Autodesk Fusion 360 part; units mm, degrees
sketch "Sketch1" plane through (0, 0, 0) normal (0, 0, 1) x (1, 0, 0)
  line L0 (0, 6.5) -> (0, -6.5) construction
  circle A0 centre (0, 6.5) radius 1.75
  circle A1 centre (0, -6.5) radius 1.75
  line L1 (4, -4.5) -> (-4, -4.5)
  line L2 (-4, -4.5) -> (-4, 4.5) construction
  line L3 (-4, 4.5) -> (4, 4.5)
  line L4 (4, 4.5) -> (4, -4.5) construction
  line L5 (4, -4.5) -> (-4, 4.5) construction
  line L6 (-4, -4.5) -> (4, 4.5) construction
  line L7 (4, -10.5) -> (-4, -10.5)
  line L8 (-4, -10.5) -> (-4, 10.5)
  line L9 (-4, 10.5) -> (4, 10.5)
  line L10 (4, 10.5) -> (4, -10.5)
  line L11 (4, -10.5) -> (-4, 10.5) construction
  line L12 (-4, -10.5) -> (4, 10.5) construction
  circle A2 centre (0, -6.5) radius 1.4
  circle A3 centre (0, 6.5) radius 1.4
  dimension "d1" = 13
  dimension "d2" = 3.5
  dimension "d3" = 3.5
  dimension "d5" = 9
  dimension "d10" = 2.8
  dimension "d11" = 2.8
  dimension "d14" = 4
  dimension "d15" = 4
extrude "Extrude1" add sketch "Sketch1" along normal blind 3.5 contours L1 L7 L8 L10 | L1 L3 L8 L10 | L3 L8 L9 L10
extrude "Extrude2" add sketch "Sketch1" along normal blind 1 contours A0 | A1
extrude "Extrude3" add sketch "Sketch1" along normal blind 10 contours L1 L3 L8 L10
sketch "Sketch2" plane through (0, -4.5, 0) normal (0, -1, 0) x (1, 0, 0)
  line L0 (-4, 3.5) -> (4, 3.5)
  line L1 (4, 3.5) -> (4, 10)
  line L2 (4, 10) -> (-4, 10)
  line L3 (-4, 10) -> (-4, 3.5)
  circle A0 centre (0, 6) radius 2.1
  line L4 (0, 6) -> (0, 3.5)
  circle A1 centre (0, 6) radius 1.6
  dimension "d18" = 4.2
  dimension "d19" = 2.5
  dimension "d24" = 3.2
extrude "Extrude4" cut sketch "Sketch2" against normal blind 14 contours A1 | A0
fillet "Fillet1" radius 3 2 edges at (-4, 0, 10) (4, 0, 10)
extrude "Extrude5" add sketch "Sketch2" against normal blind 1 contours A0
fillet "Fillet2" radius 3 4 edges at (4, -10.5, 1.75) (-4, -10.5, 1.75) (-4, 10.5, 1.75) (4, 10.5, 1.75)
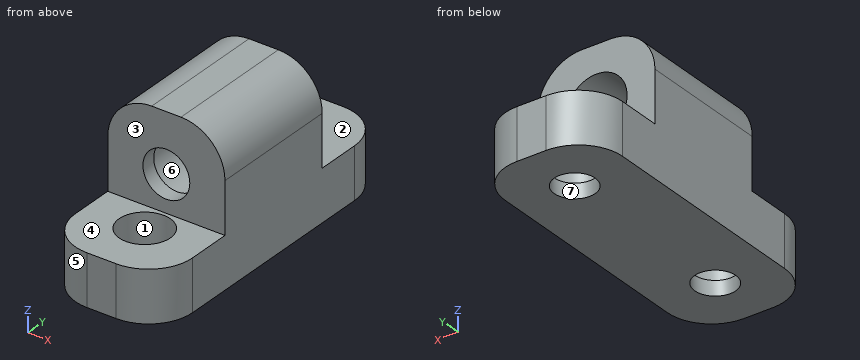
Input: part model. Units: mm. Frame: model coordinates. Face numbers are marked on the shaded views. A direction names the side the tool comes from. Give positions to 0.01 mm unless a question says otherwise; leave off trailing zeros. Order: outer loops, then holes, each group sorted by start corner. A loop starts at its lowest first (then second) coordinate and runs counter-clockwise, first axis right, second up. Notation, with made-up numbers: M 57.25,47 L 101.25,47 A9 cw 101.25,56 Z; hole C 46,15.5 d6. An arc over 180 degrees is marked long. Return JSON: item names as keys, results as strings.
Item 1: First-contact query: P1, Ø1.8, axis at x = 2, y = -7, coming from the +Z side; P2, Ø4, axis at y = 5.5, z = 5.5, coming from the -X side; P3, Ø1.5, axis at x = 3, z = 1.5, coming from the -Y side; P4, Ø2, axis at x = -1.5, z = 6.5, coming from the +Y side. Flat tips, straight axial feed; report the tip coordinate or a pass-through.
Solutions:
{"P1": "z = 3.5", "P2": "x = -4", "P3": "y = -10.23", "P4": "y = 4.5"}
Item 2: Pull-direction query (X, two-part tool) for the marked faces 4, 5, 6 and 7; classes: +X half, -X half, draft (parallel to the pull), parting line (faces both ways), or undercut.
Solutions:
{"face 4": "draft", "face 5": "-X half", "face 6": "undercut", "face 7": "undercut"}
Item 3: Cut plane B-B (y = 4.25). Return loops of the section in (x, z).
Solutions:
{"outline": "M -4,0 L 4,0 L 4,7 A3 ccw 1,10 L -1,10 A3 ccw -4,7 Z; hole C 0,6 d4.2"}
Item 4: Cut plane C-C (z = 2.5). Return loops of the section in (x, y), then the cut area to 3 significant figures.
Solutions:
{"outline": "M -4,-7.5 A3 ccw -1,-10.5 L 1,-10.5 A3 ccw 4,-7.5 L 4,7.5 A3 ccw 1,10.5 L -1,10.5 A3 ccw -4,7.5 Z; hole C 0,-6.5 d3.5; hole C 0,6.5 d3.5", "area": "141 mm^2"}
Item 5: Access query for the marked faces 1, 2 and 3. Directions: +Z, -Z, +X, -X, +Y, -Y. A direction counts if a zero-diameter tool reaches every point of the face in a straight line with its end or side. Return the directions, or none.
Solutions:
{"face 1": "+Z", "face 2": "+Z, +X, -X, +Y", "face 3": "+Z, +X, -X, -Y"}
Item 6: Cut plane A-A (x = 0). State how many separate pieces and enclosed holes the cut face has, then the cut area to 3 significant figures.
Solutions:
{"separate pieces": "4", "enclosed holes": "0", "area": "72.1 mm^2"}
Item 7: Cut plane D-D (y = 6.5). Return loops of the section in (x, z).
Solutions:
{"outline": "M -4,0 L -1.4,0 L -1.4,1 L -1.75,1 L -1.75,3.5 L -4,3.5 Z; M 1.4,0 L 4,0 L 4,3.5 L 1.75,3.5 L 1.75,1 L 1.4,1 Z"}
Item 8: Ray query, probe 1 along Y at (x, z) = (0, 0.5); probe 2 along Z at (x, y) = (0, -4.3); probe 3 along X at (y, z) = (-0.5, 6). Return the intervals inside material, ascending.
Solutions:
{"probe 1": "-10.5 to -7.9, -5.1 to 5.1, 7.9 to 10.5", "probe 2": "0 to 4.4, 7.6 to 10", "probe 3": "-4 to -2.1, 2.1 to 4"}
